For this review, use the dimensioned drawing (mm, ordinates from the lowest corner) and the shaded views. A direction names the side the tool comes from. Coordinates: 2 decimals unless noted, no trailing zeros. Loops run counter-clockwise (first coordinate to the right, second up) from the corner with the lowest first, then second, coordinate; pieces in that order, holes last. Notation, with made-up numbers: (6.25, 57.5) - (59.25, 57.5) arc R34 ccw to (59.25, 88.5) - close; hole circle Ø1 at (65.5, 58). An arc over 180 degrees is marked (long way). Answer in a Markdown table with one row per item. Add a question column.
(1) We need section B-B on z = 19. Write out the cut boundary in (x, y), plus the area to 3 significant figures.
(2) For P1, Ø4, axis at x = 19.5, z = 16, coming from the +Y side; P2, Ø5, axis at x = 4.5, y = 20, coming from the +Z side; P3, Ø3.5, axis at x = 5, z = 22.5, coming from the +Y side; P4, Ø10, axis at y = 29, z = 3, coming from the +X side, all flat-tipped, find the tip position at first contact; note any pin that passes through.
(3) We need section D-D on z = 4.5. Write out the cut boundary in (x, y), plus the area to 3 significant figures.
(4) We need section A-A on z = 8.5. Write out the cut boundary in (x, y).
(5) For line 1 along X through (y, z) = (0.5, 22.5); line 2 along Y through (x, z) = (20.5, 11.5), list the stretches that pass through material, from the lowest coordinate up.
(6) We need section C-C on x = 5. Write out the cut boundary in (y, z), plus the area to 3 significant figures.
(7) Machinability: for the marked faces 1 and 2, which of the approach directions +Z, -Z, +X, -X, +Y, -Y give a long, thin tool a straight path to every point of the face, cutting with its end or side? Answer none if there is none.
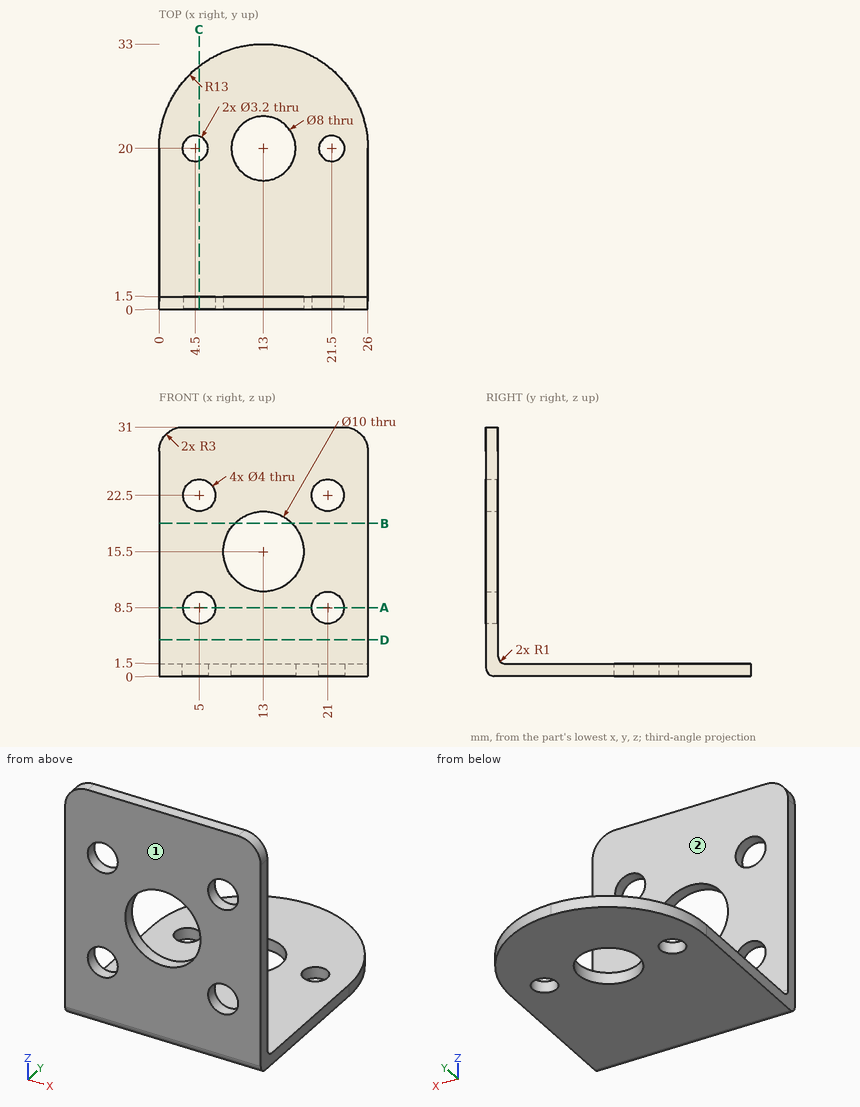
Outcome:
| question | item | result |
|---|---|---|
| 1 | outline | (0, 0) - (9.43, 0) - (9.43, 1.5) - (0, 1.5) - close; (16.57, 0) - (26, 0) - (26, 1.5) - (16.57, 1.5) - close |
| 1 | area | 28.3 mm² |
| 2 | P1 | y = 1.5 |
| 2 | P2 | z = 1.5 |
| 2 | P3 | through |
| 2 | P4 | x = 25.29 |
| 3 | outline | (0, 0) - (26, 0) - (26, 1.5) - (0, 1.5) - close |
| 3 | area | 39.0 mm² |
| 4 | outline | (0, 0) - (3, 0) - (3, 1.5) - (0, 1.5) - close; (7, 0) - (19, 0) - (19, 1.5) - (7, 1.5) - close; (23, 0) - (26, 0) - (26, 1.5) - (23, 1.5) - close |
| 5 | line 1 | 0 to 3, 7 to 19, 23 to 26 |
| 5 | line 2 | 0 to 1.5 |
| 6 | outline | (0, 1) arc R1 ccw to (1, 0) - (18.48, 0) - (18.48, 1.5) - (2.5, 1.5) arc R1 cw to (1.5, 2.5) - (1.5, 6.5) - (0, 6.5) - close; (0, 10.5) - (1.5, 10.5) - (1.5, 20.5) - (0, 20.5) - close; (0, 24.5) - (1.5, 24.5) - (1.5, 31) - (0, 31) - close; (21.52, 0) - (30.25, 0) - (30.25, 1.5) - (21.52, 1.5) - close |
| 6 | area | 73.1 mm² |
| 7 | face 1 | +Z, -Z, +X, -X, -Y |
| 7 | face 2 | +Z, +X, -X, +Y |
